```python
from build123d import *

# Parameters (mm, degrees)
SKETCH1_W               = 26
SKETCH1_H               = 100
BOSS_EXTRUDE1_DEPTH     = 13
FILLET1_R               = 10
SKETCH5_W               = 10
SKETCH5_H               = 10
SKETCH5_R               = 2.5
BOSS_EXTRUDE3_DEPTH     = 7.5
FILLET2_R               = 5
CUT_EXTRUDE1_DEPTH      = 104.431136533
CUT_EXTRUDE1_DEPTH_BACK = 104.431136533
SKETCH6_W               = 23
SKETCH6_H               = 20
CUT_EXTRUDE2_DEPTH      = 104.43113663
CUT_EXTRUDE2_DEPTH_BACK = 104.43113663
SKETCH3_R               = 4


with BuildPart() as part:
    # Sketch1 → Boss-Extrude1 (new, symmetric)
    with BuildSketch(Plane(origin=(0, 0, 0), x_dir=(0, 0, -1), z_dir=(1, 0, 0))):
        with Locations((0, 50)):
            Rectangle(SKETCH1_W, SKETCH1_H)
    extrude(amount=BOSS_EXTRUDE1_DEPTH, both=True)

    # Fillet1
    fillet1_edges = [part.edges().sort_by_distance(p)[0] for p in [
        (-13, 0, 0),
        (13, 0, 0),
    ]]
    fillet(fillet1_edges, radius=FILLET1_R)

    # Sketch5 → Boss-Extrude3 (add, symmetric)
    with BuildSketch(Plane.XY):
        with Locations((18, 90)):
            Rectangle(SKETCH5_W, SKETCH5_H)
        with Locations((18, 90)):
            Circle(SKETCH5_R, mode=Mode.SUBTRACT)
    extrude(amount=BOSS_EXTRUDE3_DEPTH, both=True)

    # Fillet2
    # the kernel refuses this fillet: 5 mm, written as the material it adds along each edge
    with BuildSketch(Plane(origin=(13, 85, 7.5), x_dir=(0, 0, 1), z_dir=(0, 1, 0))) as fillet2_piece_1_section:
        with BuildLine():
            CenterArc((FILLET2_R, FILLET2_R), FILLET2_R, 180, 90)
            Line((0, FILLET2_R), (0, 0))
            Line((0, 0), (FILLET2_R, 0))
        make_face()
    fillet2_piece_1 = extrude(amount=10, mode=Mode.PRIVATE)
    fillet2_piece_1 = fillet2_piece_1 - Plane(origin=(18, 90, 8.676026407), x_dir=(1, 0, 0), z_dir=(0, 0, -1)) * Cylinder(2.5, 41, mode=Mode.PRIVATE)
    add(fillet2_piece_1)
    with BuildSketch(Plane(origin=(13, 85, -7.5), x_dir=(0, 0, -1), z_dir=(0, 1, 0))) as fillet2_piece_2_section:
        with BuildLine():
            CenterArc((FILLET2_R, -FILLET2_R), FILLET2_R, 90, 90)
            Line((0, -FILLET2_R), (0, 0))
            Line((0, 0), (FILLET2_R, 0))
        make_face()
    fillet2_piece_2 = extrude(amount=10, mode=Mode.PRIVATE)
    fillet2_piece_2 = fillet2_piece_2 - Plane(origin=(18, 90, -8.676026407), x_dir=(1, 0, 0), z_dir=(0, 0, -1)) * Cylinder(2.5, 41, mode=Mode.PRIVATE)
    add(fillet2_piece_2)
    with BuildSketch(Plane(origin=(13, 95, -7.5), x_dir=(0, 1, 0), z_dir=(0, 0, 1))) as fillet2_piece_3:
        with BuildLine():
            CenterArc((FILLET2_R, -FILLET2_R), FILLET2_R, 90, 90)
            Line((0, -FILLET2_R), (0, 0))
            Line((0, 0), (FILLET2_R, 0))
        make_face()
    extrude(amount=15)
    with BuildSketch(Plane(origin=(13, 85, -7.5), x_dir=(0, -1, 0), z_dir=(0, 0, 1))) as fillet2_piece_4:
        with BuildLine():
            CenterArc((FILLET2_R, FILLET2_R), FILLET2_R, 180, 90)
            Line((0, FILLET2_R), (0, 0))
            Line((0, 0), (FILLET2_R, 0))
        make_face()
    extrude(amount=15)
    with BuildSketch(Plane(origin=(13, 72.5, 7.5), x_dir=(0, 0, 1), z_dir=(0, 1, 0))) as fillet2_piece_5a_section:
        with BuildLine():
            CenterArc((FILLET2_R, FILLET2_R), FILLET2_R, 180, 90)
            Line((0, FILLET2_R), (0, 0))
            Line((0, 0), (FILLET2_R, 0))
        make_face()
    fillet2_piece_5a = extrude(amount=22.5, mode=Mode.PRIVATE)
    fillet2_piece_5a = split(fillet2_piece_5a, bisect_by=Plane(origin=(14.131975571, 85, 8.631975571), z_dir=(0, -1, 0)), keep=Keep.TOP, mode=Mode.PRIVATE)
    with BuildSketch(Plane(origin=(13, 85, -7.5), x_dir=(0, -1, 0), z_dir=(0, 0, 1))) as fillet2_piece_5b_section:
        with BuildLine():
            CenterArc((FILLET2_R, FILLET2_R), FILLET2_R, 180, 90)
            Line((0, FILLET2_R), (0, 0))
            Line((0, 0), (FILLET2_R, 0))
        make_face()
    fillet2_piece_5b = extrude(amount=27.5, mode=Mode.PRIVATE)
    fillet2_piece_5b = split(fillet2_piece_5b, bisect_by=Plane(origin=(14.131975571, 83.868024429, 13), z_dir=(0, 0, -1)), keep=Keep.TOP, mode=Mode.PRIVATE)
    fillet2_piece_5b = split(fillet2_piece_5b, bisect_by=Plane(origin=(14.131975571, 83.868024429, 7.5), z_dir=(0, 0, 1)), keep=Keep.TOP, mode=Mode.PRIVATE)
    fillet2_piece_5 = fillet2_piece_5a & fillet2_piece_5b
    add(fillet2_piece_5)
    with BuildSketch(Plane(origin=(13, 95, -7.5), x_dir=(0, 1, 0), z_dir=(0, 0, 1))) as fillet2_piece_6a_section:
        with BuildLine():
            CenterArc((FILLET2_R, -FILLET2_R), FILLET2_R, 90, 90)
            Line((0, -FILLET2_R), (0, 0))
            Line((0, 0), (FILLET2_R, 0))
        make_face()
    fillet2_piece_6a = extrude(amount=27.5, mode=Mode.PRIVATE)
    fillet2_piece_6a = split(fillet2_piece_6a, bisect_by=Plane(origin=(14.131975571, 96.131975571, 13), z_dir=(0, 0, -1)), keep=Keep.TOP, mode=Mode.PRIVATE)
    fillet2_piece_6a = split(fillet2_piece_6a, bisect_by=Plane(origin=(14.131975571, 96.131975571, 7.5), z_dir=(0, 0, 1)), keep=Keep.TOP, mode=Mode.PRIVATE)
    with BuildSketch(Plane(origin=(13, 85, 7.5), x_dir=(0, 0, 1), z_dir=(0, 1, 0))) as fillet2_piece_6b_section:
        with BuildLine():
            CenterArc((FILLET2_R, FILLET2_R), FILLET2_R, 180, 90)
            Line((0, FILLET2_R), (0, 0))
            Line((0, 0), (FILLET2_R, 0))
        make_face()
    fillet2_piece_6b = extrude(amount=22.5, mode=Mode.PRIVATE)
    fillet2_piece_6b = split(fillet2_piece_6b, bisect_by=Plane(origin=(14.131975571, 100, 8.631975571), z_dir=(0, -1, 0)), keep=Keep.TOP, mode=Mode.PRIVATE)
    fillet2_piece_6b = split(fillet2_piece_6b, bisect_by=Plane(origin=(14.131975571, 95, 8.631975571), z_dir=(0, 1, 0)), keep=Keep.TOP, mode=Mode.PRIVATE)
    fillet2_piece_6 = fillet2_piece_6a & fillet2_piece_6b
    add(fillet2_piece_6)
    with BuildSketch(Plane(origin=(13, 85, -20), x_dir=(0, -1, 0), z_dir=(0, 0, 1))) as fillet2_piece_7a_section:
        with BuildLine():
            CenterArc((FILLET2_R, FILLET2_R), FILLET2_R, 180, 90)
            Line((0, FILLET2_R), (0, 0))
            Line((0, 0), (FILLET2_R, 0))
        make_face()
    fillet2_piece_7a = extrude(amount=27.5, mode=Mode.PRIVATE)
    fillet2_piece_7a = split(fillet2_piece_7a, bisect_by=Plane(origin=(14.131975571, 83.868024429, -13), z_dir=(0, 0, 1)), keep=Keep.TOP, mode=Mode.PRIVATE)
    fillet2_piece_7a = split(fillet2_piece_7a, bisect_by=Plane(origin=(14.131975571, 83.868024429, -7.5), z_dir=(0, 0, -1)), keep=Keep.TOP, mode=Mode.PRIVATE)
    with BuildSketch(Plane(origin=(13, 72.5, -7.5), x_dir=(0, 0, -1), z_dir=(0, 1, 0))) as fillet2_piece_7b_section:
        with BuildLine():
            CenterArc((FILLET2_R, -FILLET2_R), FILLET2_R, 90, 90)
            Line((0, -FILLET2_R), (0, 0))
            Line((0, 0), (FILLET2_R, 0))
        make_face()
    fillet2_piece_7b = extrude(amount=22.5, mode=Mode.PRIVATE)
    fillet2_piece_7b = split(fillet2_piece_7b, bisect_by=Plane(origin=(14.131975571, 85, -8.631975571), z_dir=(0, -1, 0)), keep=Keep.TOP, mode=Mode.PRIVATE)
    fillet2_piece_7 = fillet2_piece_7a & fillet2_piece_7b
    add(fillet2_piece_7)
    with BuildSketch(Plane(origin=(13, 95, -20), x_dir=(0, 1, 0), z_dir=(0, 0, 1))) as fillet2_piece_8a_section:
        with BuildLine():
            CenterArc((FILLET2_R, -FILLET2_R), FILLET2_R, 90, 90)
            Line((0, -FILLET2_R), (0, 0))
            Line((0, 0), (FILLET2_R, 0))
        make_face()
    fillet2_piece_8a = extrude(amount=27.5, mode=Mode.PRIVATE)
    fillet2_piece_8a = split(fillet2_piece_8a, bisect_by=Plane(origin=(14.131975571, 96.131975571, -13), z_dir=(0, 0, 1)), keep=Keep.TOP, mode=Mode.PRIVATE)
    fillet2_piece_8a = split(fillet2_piece_8a, bisect_by=Plane(origin=(14.131975571, 96.131975571, -7.5), z_dir=(0, 0, -1)), keep=Keep.TOP, mode=Mode.PRIVATE)
    with BuildSketch(Plane(origin=(13, 85, -7.5), x_dir=(0, 0, -1), z_dir=(0, 1, 0))) as fillet2_piece_8b_section:
        with BuildLine():
            CenterArc((FILLET2_R, -FILLET2_R), FILLET2_R, 90, 90)
            Line((0, -FILLET2_R), (0, 0))
            Line((0, 0), (FILLET2_R, 0))
        make_face()
    fillet2_piece_8b = extrude(amount=22.5, mode=Mode.PRIVATE)
    fillet2_piece_8b = split(fillet2_piece_8b, bisect_by=Plane(origin=(14.131975571, 100, -8.631975571), z_dir=(0, -1, 0)), keep=Keep.TOP, mode=Mode.PRIVATE)
    fillet2_piece_8b = split(fillet2_piece_8b, bisect_by=Plane(origin=(14.131975571, 95, -8.631975571), z_dir=(0, 1, 0)), keep=Keep.TOP, mode=Mode.PRIVATE)
    fillet2_piece_8 = fillet2_piece_8a & fillet2_piece_8b
    add(fillet2_piece_8)
    # the kernel refuses this fillet: 5 mm, written as the material it takes off along each edge
    with BuildSketch(Plane(origin=(23, 107.5, -7.5), x_dir=(-1, 0, 0), z_dir=(0, -1, 0)), Plane(origin=(23, 107.5, 7.5), x_dir=(0, 0, -1), z_dir=(0, -1, 0))) as fillet2_2_piece_1:
        with BuildLine():
            CenterArc((FILLET2_R, -FILLET2_R), FILLET2_R, 90, 90)
            Line((0, -FILLET2_R), (0, 0))
            Line((0, 0), (FILLET2_R, 0))
        make_face()
    extrude(amount=35, mode=Mode.SUBTRACT)
    with BuildSketch(Plane(origin=(23, 95, 20), x_dir=(-1, 0, 0), z_dir=(0, 0, -1)), Plane(origin=(23, 85, 20), x_dir=(0, 1, 0), z_dir=(0, 0, -1))) as fillet2_2_piece_2:
        with BuildLine():
            CenterArc((FILLET2_R, -FILLET2_R), FILLET2_R, 90, 90)
            Line((0, -FILLET2_R), (0, 0))
            Line((0, 0), (FILLET2_R, 0))
        make_face()
    extrude(amount=40, mode=Mode.SUBTRACT)

    # Sketch6 → Cut-Extrude1 (cut, two sides: drawn at the far end of the back side and taken through both)
    with BuildSketch(Plane(origin=(0, 100, 0), x_dir=(1, 0, 0), z_dir=(0, 1, 0)).offset(-CUT_EXTRUDE1_DEPTH_BACK)):
        with Locations((-1.5, 0)):
            Rectangle(SKETCH6_W, SKETCH6_H)
    extrude(amount=CUT_EXTRUDE1_DEPTH + CUT_EXTRUDE1_DEPTH_BACK, mode=Mode.SUBTRACT)

    # Sketch3 → Cut-Extrude2 (cut, two sides: drawn at the far end of the back side and taken through both)
    with BuildSketch(Plane.XY.offset(-CUT_EXTRUDE2_DEPTH_BACK)):
        with Locations((0, 11)):
            Circle(SKETCH3_R)
        with Locations((0, 89)):
            Circle(SKETCH3_R)
    extrude(amount=CUT_EXTRUDE2_DEPTH + CUT_EXTRUDE2_DEPTH_BACK, mode=Mode.SUBTRACT)


solid = part.part
```
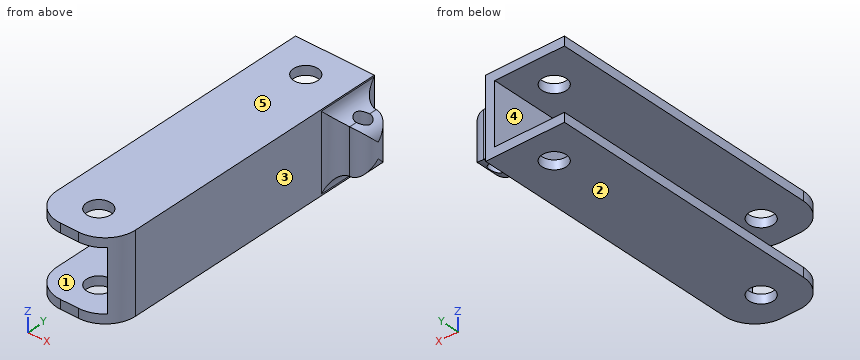
CAD build for the part. Positions are in the model's coordinates, mm. Face numbers are marked on the shaded views. A direction names the side the tool comes from. Round coordinates to 2 decimals unless told otherwise and drop trailing zeros. Order: outer loops, then holes, each group sorted by start corner. A loop starts at its lowest first (then second) coordinate and runs counter-clockwise, first axis right, second up.
Item 1: Saw through at C-C on x = 0. Write the cut outline in (y, z).
Item 2: Probe line 1 along Y through (x, z) = (0, -11.7); line 2 along Z through (x, y) = (9, 19.5); line 3 along X through (y, z) = (11, 10.65). List the from-to ranges inside material, lowest first.
Item 3: Saw through at B-B on y = 11. Write the cut outline in (x, z), then the cut area to 3 significant figures.
Item 4: Tool access for the marked faces 1 and 2: list every direction of +Z, -Z, +X, -X, +Y, -Y with a clear straight run to the whole face (end or side of a thin tool).
Item 5: Saw through at A-A on x = -10. Write the cut outline in (y, z), then the cut area to 3 significant figures.
Item 6: Saw through at D-D on y = 89. Write the cut outline in (x, z), then the cut area to 3 significant figures.
Item 7: Mould opens along Z. For the marked faces 3, 4 and 5 say: pulls with the +Z half, pulls with the -Z half, needs draft (parallel to the pull), parting line crosses it, or undercut.
Item 8: Pin check, flat tips, straight feed: pin 1 (8 mm diameter, centred on y = 63, z = 5.5, fed in from +X); pin 2 (1.5 mm diameter, centred on x = -2.5, y = 88, fed in from +Z); pin 3 (13 mm diameter, centred on x = 0, y = 89, fed in from -Z). Stop position of each tip, or through.
Reported:
1. outline: (0, -13) - (7, -13) - (7, -10) - (0, -10) - close; (0, 10) - (7, 10) - (7, 13) - (0, 13) - close; (15, -13) - (85, -13) - (85, -10) - (15, -10) - close; (15, 10) - (85, 10) - (85, 13) - (15, 13) - close; (93, -13) - (100, -13) - (100, -10) - (93, -10) - close; (93, 10) - (100, 10) - (100, 13) - (93, 13) - close
2. line 1: y = 0 to 7, 15 to 85, 93 to 100
2. line 2: z = -13 to -10, 10 to 13
2. line 3: x = -13 to -4, 4 to 13
3. outline: (-13, -13) - (-4, -13) - (-4, -10) - (-13, -10) - close; (-13, 10) - (-4, 10) - (-4, 13) - (-13, 13) - close; (4, -13) - (13, -13) - (13, 13) - (4, 13) - (4, 10) - (10, 10) - (10, -10) - (4, -10) - close
3. area: 168 mm2
4. face 1: -X, +Y, -Y
4. face 2: -Z, +X, -X, +Y, -Y
5. outline: (2.86, -13) - (100, -13) - (100, -10) - (2.86, -10) - close; (2.86, 10) - (100, 10) - (100, 13) - (2.86, 13) - close
5. area: 583 mm2
6. outline: (-13, -13) - (-4, -13) - (-4, -10) - (-13, -10) - close; (-13, 10) - (-4, 10) - (-4, 13) - (-13, 13) - close; (4, -13) - (13, -13) - (13, -12.5) arc R5 cw to (15.71, -8.06) - (15.71, 8.06) arc R5 cw to (13, 12.5) - (13, 13) - (4, 13) - (4, 10) - (10, 10) - (10, -10) - (4, -10) - close; (20.29, -6.94) arc R5 ccw to (22.9, -3.5) - (22.9, 3.5) arc R5 ccw to (20.29, 6.94) - close
6. area: 249 mm2
7. face 3: needs draft
7. face 4: undercut
7. face 5: pulls with the +Z half
8. pin 1: stops at x = 13
8. pin 2: passes through
8. pin 3: stops at z = -13
